Answer from the drawing. Dimensions are ordinates in mm from the lowest x, y and z of the part. Give positions to 0.01 mm unless a question says otherwise; leave off trailing zeros. Order: outer loops, then holes, each group sorted by start corner. A loop starts at its lowest first (then second) coordinate and runs counter-clockwise, first axis right, second up.
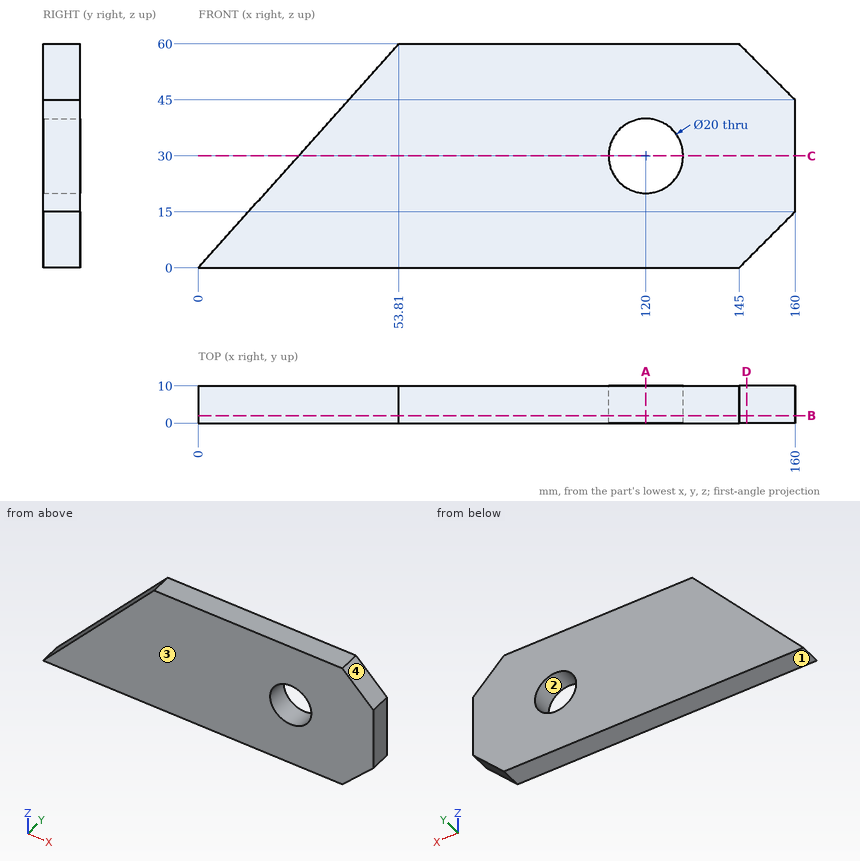
1) For a pull along Z with two mould halves and no side action, classify the marked faces 1, 2, 3 and 4 as released by +Z, released by -Z, zero draft, split by the parting line, or undercut.
Final values:
face 1: released by -Z
face 2: undercut
face 3: zero draft
face 4: released by +Z
2) Given pin 1 (1 mm diameter, centred on x = 122, y = 4, fed in from -Z); pin 2 (1.5 mm diameter, centred on y = 3.5, z = 37.5, fed in from -X), each flat-ended and moving along its own axis, determine where each tip first touches the part or whether it passes through.
Final values:
pin 1: stops at z = 0
pin 2: stops at x = 32.96
3) The part is cut by section A-A on x = 120. Determine the outline of the cut face in (y, z).
Final values:
outline: (0, 0) - (10, 0) - (10, 20) - (0, 20) - close; (0, 40) - (10, 40) - (10, 60) - (0, 60) - close
4) The part is cut by section B-B on y = 2. Determine the outline of the cut face in (x, z).
Final values:
outline: (0, 0) - (145, 0) - (160, 15) - (160, 45) - (145, 60) - (53.81, 60) - close; hole circle Ø20 at (120, 30)
5) The part is cut by section C-C on z = 30. Determine the outline of the cut face in (x, y) (1 decimal).
Final values:
outline: (26.9, 0) - (110, 0) - (110, 10) - (26.9, 10) - close; (130, 0) - (160, 0) - (160, 10) - (130, 10) - close
6) Consider L1, parallel to Z at x = 120, y = 4; L2, parallel to X at y = 6.75, z = 22; L3, parallel to X at y = 2, z = 25.5. Determine where each line is inside the solid, lowest interval first.
Final values:
L1: z = 0 to 20, 40 to 60
L2: x = 19.73 to 114, 126 to 160
L3: x = 22.87 to 111.07, 128.93 to 160
7) The part is cut by section D-D on x = 147. Determine the outline of the cut face in (y, z).
Final values:
outline: (0, 2) - (10, 2) - (10, 58) - (0, 58) - close
